Read the model definition and answer for the solid it produces. Units are mm, in the model's axes. Face numbers are marked on the shaded views. Coordinates: 2 decimals unless noted, no trailing zeros. Order: outer loops, then holes, each group sorted by start corner. A loop starts at its lowest first (then second) coordinate and runs counter-clockwise, first axis right, second up. Notation, with made-up numbers: M 47,-23 L 78,-23 A28 cw 78,14 Z; hole C 30,71.25 d10. An arc over 180 degrees is marked long. Put each result on its own line as item: value.
from build123d import *

# Parameters (mm, degrees)
EXTRUDE1_DEPTH       = 2.794
HOLE1_D              = 1.60274
EXTRUDE2_DEPTH       = 2.794
LPATTERN1_COUNT      = 6
LPATTERN1_PITCH      = 2.54
LPATTERN1_COUNT_DIR2 = 2
LPATTERN1_PITCH_DIR2 = 2.54
LPATTERN2_COUNT      = 35
LPATTERN2_PITCH      = 2.54


with BuildPart() as part:
    # Sketch1 → Extrude1 (new body)
    with BuildSketch(Plane(origin=(0, 0, 0), x_dir=(1, 0, 0), z_dir=(0, 1, 0))):
        Polygon((14.934373708, 0.40005), (14.774353708, 0.40005), (14.628747416, 0), (0, 0), (-0.145606292, 0.40005), (-0.305626292, 0.40005), (-0.305626292, 4.67995), (-0.145606292, 4.67995), (0, 5.08), (14.628747416, 5.08), (14.774353708, 4.67995), (14.934373708, 4.67995), align=None)
    extrude(amount=-EXTRUDE1_DEPTH)

    # Hole1 (through all)
    with Locations(Plane(origin=(0.964373708, 0, -1.27), x_dir=(0, 0, 1), z_dir=(0, 1, 0))):
        with Locations((0, 0)):
            hole1 = Hole(HOLE1_D / 2)

    # Sketch4 → Extrude2 (cut)
    with BuildSketch(Plane(origin=(0, 0, 0), x_dir=(1, 0, 0), z_dir=(0, 1, 0))):
        Polygon((1.928772816, 0), (2.5399746, 0), (2.394368308, 0.40005), (2.074379108, 0.40005), align=None)
        Polygon((2.074379108, 4.67995), (2.394368308, 4.67995), (2.5399746, 5.08), (1.928772816, 5.08), align=None)
    extrude2 = extrude(amount=-EXTRUDE2_DEPTH, mode=Mode.SUBTRACT)

    # LPattern1: Hole1 6 × 2
    with Locations(*[(i * LPATTERN1_PITCH, 0, -j * LPATTERN1_PITCH_DIR2) for i in range(LPATTERN1_COUNT) for j in range(LPATTERN1_COUNT_DIR2) if (i, j) != (0, 0)]):
        add(hole1, mode=Mode.SUBTRACT)

    # LPattern2: Extrude2 ×35
    with Locations(*[(i * LPATTERN2_PITCH, 0, 0) for i in range(1, LPATTERN2_COUNT)]):
        add(extrude2, mode=Mode.SUBTRACT)


solid = part.part
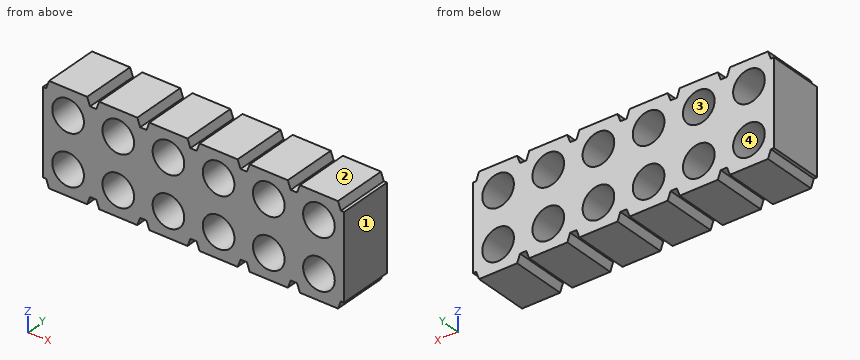
Q1. Consider line 1 along Z through (x, y) = (3.5, -1.45); line 2 along Z through (x, y) = (3.75, -0.7). Determine where each line is inside the solid, lowest interval first.
Answers below:
line 1: z = -5.08 to -4.61, -3.01 to -2.07, -0.47 to 0
line 2: z = -5.08 to -4.57, -3.05 to -2.03, -0.51 to 0
Q2. For a pull along X with two mould halves and no side action, classify the marked faces 1, 2, 3 and 4 as +X half, -X half, draft (parallel to the pull), parting line (faces both ways), or undercut.
Answers below:
face 1: +X half
face 2: draft
face 3: undercut
face 4: undercut
Q3. Find section D-D on x = 10.75. Write down the section's boundary in (y, z).
Answers below:
outline: M -2.79,-5.08 L 0,-5.08 L 0,-4.52 L -2.79,-4.52 Z; M -2.79,-3.1 L 0,-3.1 L 0,-1.98 L -2.79,-1.98 Z; M -2.79,-0.56 L 0,-0.56 L 0,0 L -2.79,0 Z
Q4. Given pin 1 (2.5 mm diameter, centred on x = 0.96, z = -3.81, fed in from +Y), flat-ended and moving along its own axis, determine where the tip first touches the part or whether it passes through.
Answers below:
pin 1: stops at y = 0
Q5. Find section B-B on x = 4. Write down the section's boundary in (y, z), plus the area to 3 significant figures.
Answers below:
outline: M -2.79,-5.08 L 0,-5.08 L 0,-4.44 L -2.79,-4.44 Z; M -2.79,-3.18 L 0,-3.18 L 0,-1.9 L -2.79,-1.9 Z; M -2.79,-0.64 L 0,-0.64 L 0,0 L -2.79,0 Z
area: 7.16 mm^2
Q6. Find section C-C on z = -3.9. Write down the section's boundary in (x, y), plus the area to 3 significant figures.
Answers below:
outline: M -0.31,-2.79 L 0.17,-2.79 L 0.17,0 L -0.31,0 Z; M 1.76,-2.79 L 2.71,-2.79 L 2.71,0 L 1.76,0 Z; M 4.3,-2.79 L 5.25,-2.79 L 5.25,0 L 4.3,0 Z; M 6.84,-2.79 L 7.79,-2.79 L 7.79,0 L 6.84,0 Z; M 9.38,-2.79 L 10.33,-2.79 L 10.33,0 L 9.38,0 Z; M 11.92,-2.79 L 12.87,-2.79 L 12.87,0 L 11.92,0 Z; M 14.46,-2.79 L 14.93,-2.79 L 14.93,0 L 14.46,0 Z
area: 15.9 mm^2
Q7. Find section A-A on z = -1.27. Write down the section's boundary in (x, y), plus the area to 3 significant figures.
Answers below:
outline: M -0.31,-2.79 L 0.16,-2.79 L 0.16,0 L -0.31,0 Z; M 1.77,-2.79 L 2.7,-2.79 L 2.7,0 L 1.77,0 Z; M 4.31,-2.79 L 5.24,-2.79 L 5.24,0 L 4.31,0 Z; M 6.85,-2.79 L 7.78,-2.79 L 7.78,0 L 6.85,0 Z; M 9.39,-2.79 L 10.32,-2.79 L 10.32,0 L 9.39,0 Z; M 11.93,-2.79 L 12.86,-2.79 L 12.86,0 L 11.93,0 Z; M 14.47,-2.79 L 14.93,-2.79 L 14.93,0 L 14.47,0 Z
area: 15.7 mm^2
